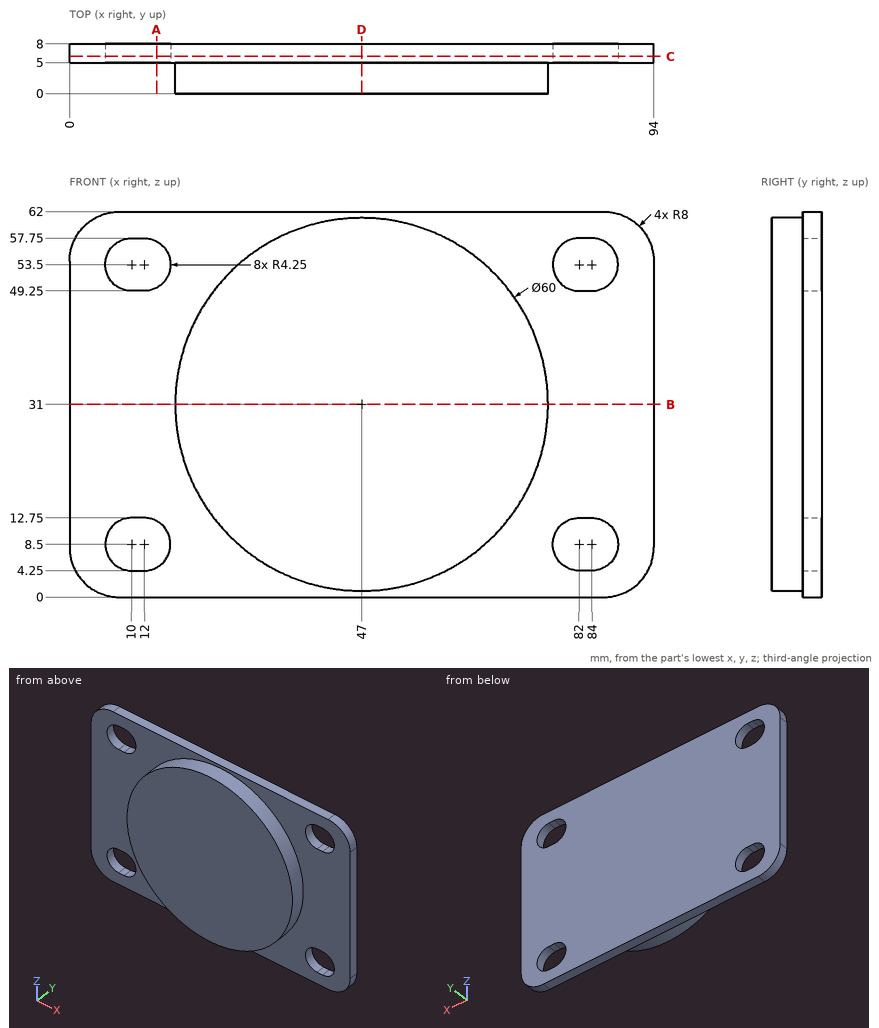
Source: three-view drawing plus pictorial views. Frame: mm from the lowest corner of the part. Coordinates: 2 decimals unless noted, no trailing zeros. Order: outer loops, then holes, each group sorted by start corner. A loop starts at its lowest first (then second) coordinate and runs counter-clockwise, first axis right, second up. Notation, with made-up numbers: M -5.75,7.5 L 50.25,7.5 A14 ccw 50.25,24.5 Z; hole C 29,-16.5 d11. An arc over 180 degrees is marked long. One line per question, with ' | ' between items.
Item 1: Pin query (flat end, axial travel): pin 1 (2 mm diameter, centred on x = 83.5, y = 6, fed in from -Z); pin 2 (1.5 mm diameter, centred on x = 27, y = 3, fed in from -Z). Return the tip coordinate at first contact, or that it passes through.
Geometry results:
pin 1: stops at z = 0 | pin 2: stops at z = 7.99
Item 2: Section C-C (y = 6). Output: boundary loops of the cut face in (x, z), then the cut area to 3 significant figures.
Geometry results:
outline: M 0,8 A8 ccw 8,0 L 86,0 A8 ccw 94,8 L 94,54 A8 ccw 86,62 L 8,62 A8 ccw 0,54 Z; hole M 10,4.25 L 12,4.25 A4.25 ccw 12,12.75 L 10,12.75 A4.25 ccw Z; hole M 10,49.25 L 12,49.25 A4.25 ccw 12,57.75 L 10,57.75 A4.25 ccw Z; hole M 82,4.25 L 84,4.25 A4.25 ccw 84,12.75 L 82,12.75 A4.25 ccw Z; hole M 82,49.25 L 84,49.25 A4.25 ccw 84,57.75 L 82,57.75 A4.25 ccw Z | area: 5,480 mm^2
Item 3: Section D-D (x = 47). Output: boundary loops of the cut face in (y, z).
Geometry results:
outline: M 0,1 L 5,1 L 5,0 L 8,0 L 8,62 L 5,62 L 5,61 L 0,61 Z
Item 4: Section A-A (x = 14). Output: boundary loops of the cut face in (y, z).
Geometry results:
outline: M 5,0 L 8,0 L 8,4.75 L 5,4.75 Z; M 5,12.25 L 8,12.25 L 8,49.75 L 5,49.75 Z; M 5,57.25 L 8,57.25 L 8,62 L 5,62 Z
Item 5: Ray query, line 1 along X through (y, z) = (7, 50.5); line 2 along X through (y, z) = (6.5, 56); line 3 along Y through (x, z) = (19, 44). Return the intervals inside material, ascending.
Geometry results:
line 1: x = 0 to 6.99, 15.01 to 78.99, 87.01 to 94 | line 2: x = 0.25 to 6.56, 15.44 to 78.56, 87.44 to 93.75 | line 3: y = 5 to 8
Item 6: Section B-B (z = 31). Output: boundary loops of the cut face in (x, y).
Geometry results:
outline: M 0,5 L 17,5 L 17,0 L 77,0 L 77,5 L 94,5 L 94,8 L 0,8 Z
